Could you check a few things on this model? Use its own coordinates, in mm. Face numbers are marked on the shaded views. A direction names the side the tool comes from. Give positions to 0.01 mm unless a question says otherwise; leave off trailing zeros. Loops run counter-clockwise (first coordinate to the right, second up) from the corner with the lowest first, then second, coordinate; pieces in that order, holes last.
1. For the marked faces 1 and 2, which set-ups out of +Z, -Z, +X, -X, +Y, -Y let a thin tool reach every point of the face, with its end or its side?
2. Imagine slicing it at A-A (y = -12.7). Count the separate pieces of the cut face and the enclosed holes in it, plus the area to 3 significant figures.
3. I need wall thicknesses on line 1 along Y through (x, z) = (-187.5, 4.5); line 2 along X through (y, z) = (-17, 5.5); line 3 along Z through (x, y) = (-141.5, -18.5) (3 decimals). Which ranges of each line are inside material? Lowest first, please.
4. For P1, Ø7.5, axis at x = -12.7, y = -12.7, coming from the +Z side; P2, Ø6, axis at x = -44.5, y = -12, coming from the +Z side (3 decimals); P3, Ø1, axis at y = -7.5, z = 5.5, coming from the +X side, each with a flat end and sliding along its axis, tell me the tip position at first contact or that it passes through.
5. Imagine slicing it at B-B (x = -98). List the corners of the cut face in (y, z) for me (3 decimals).
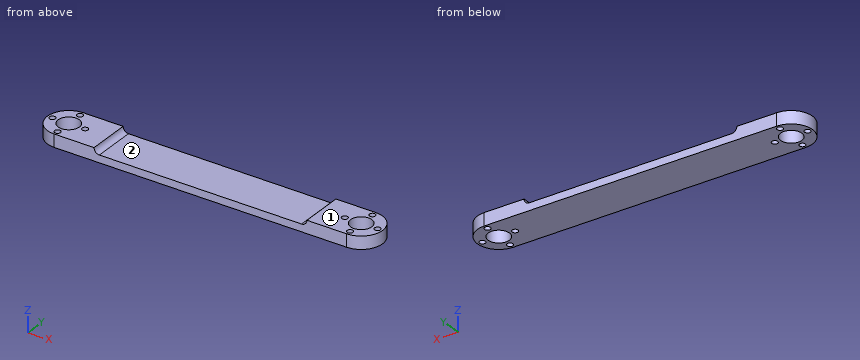
```python
from build123d import *

# Parameters (mm, degrees)
SKETCH1_R               = 12.7
BOSS_EXTRUDE1_DEPTH     = 7.62
SKETCH2_R               = 6.35
CUT_EXTRUDE1_DEPTH      = 7.62
SKETCH3_R               = 1.778
CUT_EXTRUDE2_DEPTH      = 7.62
CIRPATTERN1_COUNT       = 4
MIRROR1_COPY_1_SKETCH_R = 1.778
MIRROR1_COPY_1_DEPTH    = 7.62
MIRROR1_COPY_2_SKETCH_R = 1.778
MIRROR1_COPY_2_DEPTH    = 7.62
MIRROR1_COPY_3_SKETCH_R = 1.778
MIRROR1_COPY_3_DEPTH    = 7.62
SKETCH4_W               = 127
SKETCH4_H               = 3.175
CUT_EXTRUDE3_DEPTH      = 25.4
FILLET1_R               = 3.175


with BuildPart() as part:
    # Sketch1 → Boss-Extrude1 (new body)
    with BuildSketch(Plane.XY):
        with BuildLine():
            ThreePointArc((-12.7, -25.4), (-25.4, -12.7), (-12.7, 0))
            Line((-12.7, 0), (-187.198, 0))
            ThreePointArc((-187.198, 0), (-178.217743879, -3.719743879), (-174.498, -12.7))
            ThreePointArc((-174.498, -12.7), (-178.217743879, -21.680256121), (-187.198, -25.4))
            Line((-187.198, -25.4), (-12.7, -25.4))
        make_face()
        with Locations((-187.198, -12.7)):
            Circle(SKETCH1_R)
        with Locations((-12.7, -12.7)):
            Circle(SKETCH1_R)
    extrude(amount=BOSS_EXTRUDE1_DEPTH)

    # Sketch2 → Cut-Extrude1 (cut)
    with BuildSketch(Plane.XY.offset(7.62)):
        with Locations((-12.7, -12.7)):
            Circle(SKETCH2_R)
    cut_extrude1 = extrude(amount=-CUT_EXTRUDE1_DEPTH, mode=Mode.SUBTRACT)

    # Sketch3 → Cut-Extrude2 (cut)
    with BuildSketch(Plane.XY.offset(7.62)):
        with Locations((-2.921, -12.7)):
            Circle(SKETCH3_R)
    cut_extrude2 = extrude(amount=-CUT_EXTRUDE2_DEPTH, mode=Mode.SUBTRACT)

    # CirPattern1: Cut-Extrude2 ×4 about axis
    cirpattern1_axis = Axis((-12.7, -12.7, 0), (0, 0, 1))
    for i in range(1, CIRPATTERN1_COUNT):
        add(cut_extrude2.rotate(cirpattern1_axis, i * 360 / CIRPATTERN1_COUNT), mode=Mode.SUBTRACT)

    # Mirror1: Cut-Extrude1, Cut-Extrude2 across plane
    add(cut_extrude1.mirror(Plane(origin=(-99.949, 0, 0), x_dir=(0, 0, 1), z_dir=(1, 0, 0))), mode=Mode.SUBTRACT)
    add(cut_extrude2.mirror(Plane(origin=(-99.949, 0, 0), x_dir=(0, 0, 1), z_dir=(1, 0, 0))), mode=Mode.SUBTRACT)

    # Mirror1 copy 1 sketch → Mirror1 copy 1 (cut)
    with BuildSketch(Plane(origin=(-174.498, 0, 7.62), x_dir=(0, 1, 0), z_dir=(0, 0, 1))):
        with Locations((-2.921, 12.7)):
            Circle(MIRROR1_COPY_1_SKETCH_R)
    extrude(amount=-MIRROR1_COPY_1_DEPTH, mode=Mode.SUBTRACT)

    # Mirror1 copy 2 sketch → Mirror1 copy 2 (cut)
    with BuildSketch(Plane(origin=(-174.498, -25.4, 7.62), x_dir=(1, 0, 0), z_dir=(0, 0, 1))):
        with Locations((-2.921, 12.7)):
            Circle(MIRROR1_COPY_2_SKETCH_R)
    extrude(amount=-MIRROR1_COPY_2_DEPTH, mode=Mode.SUBTRACT)

    # Mirror1 copy 3 sketch → Mirror1 copy 3 (cut)
    with BuildSketch(Plane(origin=(-199.898, -25.4, 7.62), x_dir=(0, -1, 0), z_dir=(0, 0, 1))):
        with Locations((-2.921, 12.7)):
            Circle(MIRROR1_COPY_3_SKETCH_R)
    extrude(amount=-MIRROR1_COPY_3_DEPTH, mode=Mode.SUBTRACT)

    # Sketch4 → Cut-Extrude3 (cut)
    with BuildSketch(Plane.XZ.offset(25.4)):
        with Locations((-99.949, 6.0325)):
            Rectangle(SKETCH4_W, SKETCH4_H)
    extrude(amount=-CUT_EXTRUDE3_DEPTH, mode=Mode.SUBTRACT)

    # Fillet1
    fillet1_edges = [part.edges().sort_by_distance(p)[0] for p in [
        (-36.449, -12.7, 4.445),
        (-163.449, -12.7, 4.445),
    ]]
    fillet(fillet1_edges, radius=FILLET1_R - 0.0001)  # a hair under: the kernel refuses the full size


solid = part.part
```
Derived:
1. face 1: +Z, +X, -X, +Y, -Y
1. face 2: +Z, +Y, -Y
2. separate pieces: 7
2. enclosed holes: 0
2. area: 822 mm2
3. line 1: y = -25.4 to -24.23, -20.73 to -19.04, -6.36 to -4.67, -1.17 to 0
3. line 2: x = -199.15 to -191.87, -182.53 to -162.64, -37.26 to -17.37, -8.03 to -0.75
3. line 3: z = 0 to 4.445
4. P1: passes through
4. P2: stops at z = 4.445
4. P3: stops at x = -0.9
5. outline: (-25.4, 0) - (0, 0) - (0, 4.445) - (-25.4, 4.445) - close
